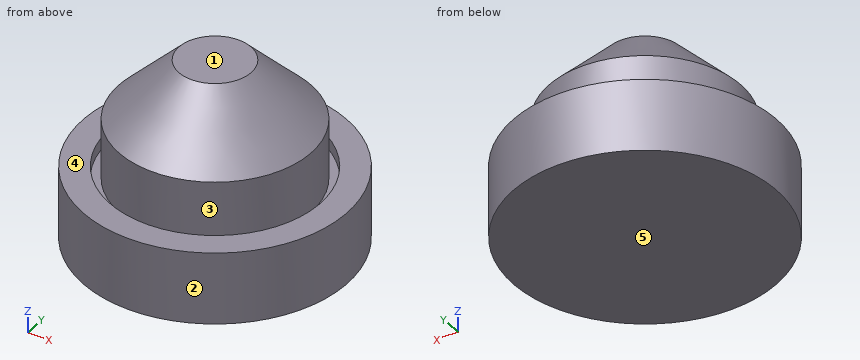
```python
from build123d import *

# Parameters (mm, degrees)
F0_R     = 55.878633
F1_DEPTH = 25.4
F2_R     = 55.878633
F2_R_2   = 44.572454
F4_DEPTH = 5.08
F3_R     = 40.718118
F5_DEPTH = 50.8
F6_SIZE  = 25.4


with BuildPart() as f1:
    # F0 (on Top) → F1 (new body)
    with BuildSketch(Plane.XY):
        Circle(F0_R)
    extrude(amount=F1_DEPTH)

    # F2 (on face) → F4 (join)
    with BuildSketch(Plane.XY.offset(25.4)):
        Circle(F2_R)
        Circle(F2_R_2, mode=Mode.SUBTRACT)
    extrude(amount=F4_DEPTH)

    # F3 (on face) → F5 (join)
    with BuildSketch(Plane.XY.offset(25.4)):
        Circle(F3_R)
    extrude(amount=F5_DEPTH)

    # F6
    f6_edges = [f1.edges().sort_by_distance(p)[0] for p in [
        (-40.718118, 0, 76.2),
    ]]
    chamfer(f6_edges, length=F6_SIZE)


solid = f1.part
```
Part model, mm, in its own coordinate system. Face numbers are marked on the shaded views. A direction names the side the tool comes from. Coordinates: 2 decimals unless noted, no trailing zeros. Loops run counter-clockwise (first coordinate to the right, second up) from the corner with the lowest first, then second, coordinate; pieces in that order, holes last. Notation, with made-up numbers: (64, 67) - (68, 67) arc R19 ccw to (68, 90) - close; hole circle Ø8 at (27.25, 82). An arc over 180 degrees is marked (long way). Write item = value, one per line. Start each with the question number.
Item 1: 3-axis set-ups, long thin cutter, end or side, ignore diameter. For the marked faces 4 and 5: which of +Z, -Z, +X, -X, +Y, -Y reach the whole face in a straight line?
Item 2: Cut at A-A, the plane x = 0. Give the cut face in (y, z), and give its area (3 significant figures).
Item 3: Mould opens along Y. For the marked faces 1, 2 and 3 say: released by +Y, released by -Y, zero draft, split by the parting line, or undercut.
Item 4: Flat gauge pins, fed straight in: pin 1 Ø3 at (y, z) = (38.5, 29.5) entering from +X; pin 2 Ø10 at (x, z) = (9.5, 30.5) entering from +Y; pin 3 Ø2 at (x, y) = (-35, 11) entering from -Z; pin 4 Ø2 at (x, z) = (5, 17) entering from -Y. Where does each tip first touch, or does it go through?
Item 5: Wall check: L1, parallel to Y at x = 0, z = 28; L2, parallel to X at y = 35.5, z = 27; L3, parallel to Z at x = 17, y = -50. Give the ranges that are in metal, low to high. Write a range as from..to.
Item 6: Cut at C-C, the plane z = 17.5. Give the cut face in (x, y).
Item 7: Cut at D-D, the plane x = 49.5. Give the cut face in (y, z), and give its area (3 significant figures).
The answers:
q1.face_4 = +Z
q1.face_5 = -Z, +X, -X, +Y, -Y
q2.outline = (-55.88, 0) - (55.88, 0) - (55.88, 30.48) - (44.57, 30.48) - (44.57, 25.4) - (40.72, 25.4) - (40.72, 50.8) - (15.32, 76.2) - (-15.32, 76.2) - (-40.72, 50.8) - (-40.72, 25.4) - (-44.57, 25.4) - (-44.57, 30.48) - (-55.88, 30.48) - close
q2.area = 6,450 mm2
q3.face_1 = zero draft
q3.face_2 = split by the parting line
q3.face_3 = undercut
q4.pin_1 = 41.87
q4.pin_2 = 55.7
q4.pin_3 = 0
q4.pin_4 = -55.74
q5.L1 = -55.88..-44.57, -40.72..40.72, 44.57..55.88
q5.L2 = -43.15..-26.95, -19.94..19.94, 26.95..43.15
q5.L3 = 0..30.48
q6.outline = circle Ø111.76 at (0, 0)
q7.outline = (-25.93, 0) - (25.93, 0) - (25.93, 30.48) - (-25.93, 30.48) - close
q7.area = 1,580 mm2
